```python
from build123d import *

# Parameters (mm, degrees)
Y_KSEKLIK_EKSTR_ZYON1_DEPTH = 3
Y_KSEKLIK_EKSTR_ZYON3_DEPTH = 15.352247347
KES_EKSTR_ZYON6_DEPTH       = 83.869457244
RADYUS1_R                   = 1
IZIM9_R                     = 2.8
KES_EKSTR_ZYON7_DEPTH       = 13


with BuildPart() as part:
    # Çizim1 → Yükseklik-Ekstrüzyon1 (new body)
    with BuildSketch(Plane.XY):
        with BuildLine():
            Line((51.744165627, 14.308045798), (56.895737739, 14.308045798))
            Line((56.895737739, 14.308045798), (56.895737739, 29.660293145))
            Line((56.895737739, 29.660293145), (-67.032214562, 29.660293145))
            Line((-67.032214562, 29.660293145), (-67.032214562, -18.6200596))
            add(Edge.make_bspline(
                [(51.744165627, 14.308045798), (32.353014477, 13.942055171), (-5.53549701, 3.029288221), (-42.761336594, -18.994069798), (-67.032214562, -18.6200596)],
                knots=[0, 0, 0, 0, 0.428556307, 1, 1, 1, 1], degree=3))
        make_face()
    extrude(amount=Y_KSEKLIK_EKSTR_ZYON1_DEPTH)

    # Çizim5 → Yükseklik-Ekstrüzyon3 (add)
    with BuildSketch(Plane(origin=(0, 29.660293145, 0), x_dir=(1, 0, 0), z_dir=(0, 1, 0))):
        with BuildLine():
            Line((57.574880058, 1.015986664), (56.895737739, 0))
            Line((56.895737739, 0), (56.895737739, -3))
            Line((56.895737739, -3), (57.574880058, -4.015986664))
            Line((57.574880058, -4.015986664), (57.918910072, -4.530650376))
            ThreePointArc((57.918910072, -4.530650376), (66.895737739, -1.5), (57.918910072, 1.530650376))
            Line((57.918910072, 1.530650376), (57.574880058, 1.015986664))
        make_face()
    extrude(amount=-Y_KSEKLIK_EKSTR_ZYON3_DEPTH)

    # Çizim7 → Kes-Ekstrüzyon6 (cut, through all)
    with BuildSketch(Plane(origin=(0, 29.660293145, 0), x_dir=(1, 0, 0), z_dir=(0, 1, 0))):
        Polygon((-67.032214562, -0.5), (56.895737739, 0), (-67.032214562, 0), align=None)
        Polygon((-67.032214562, -3), (56.895737739, -3), (-67.032214562, -2.5), align=None)
    extrude(amount=-KES_EKSTR_ZYON6_DEPTH, mode=Mode.SUBTRACT)

    # Radyus1
    radyus1_edges = [part.edges().sort_by_distance(p)[0] for p in [
        (-67.032214562, 5.520116772, 2.5),
        (-67.032214562, 5.520116772, 0.5),
    ]]
    fillet(radyus1_edges, radius=RADYUS1_R)

    # Çizim9 → Kes-Ekstrüzyon7 (cut)
    with BuildSketch(Plane(origin=(0, 29.660293145, 0), x_dir=(-1, 0, 0), z_dir=(0, 1, 0))):
        with Locations(Location((-61.895737739, 1.5, 0), (0, 0, 90))):
            Circle(IZIM9_R)
    extrude(amount=-KES_EKSTR_ZYON7_DEPTH, mode=Mode.SUBTRACT)


solid = part.part
```
For this review, take the finished solid that the model builds, in its own axes (mm). A direction names the side the tool comes from. Round coordinates to 2 decimals unless told otherwise and drop trailing zeros. One line per item, written item: value. Start each with the question number.
(1) Insertion check: pin 1 (1.5 mm diameter, centred on x = -4, y = 15.5, fed in from +Z); pin 2 (8 mm diameter, centred on x = -30, y = -6.5, fed in from +Z); pin 3 (1.5 mm diameter, centred on y = 23.5, z = 4.5, fed in from -X). Each pin has a flat end and moves straight along its axis. Give the tip position at first contact, or say it passes through.
(2) Machinability: for faces 1 (the flat face through (61, 14.308, 1)), 2 (the cylindrical face through (64.257, 23.251, 3.005)), which of the approach directions +Z, -Z, +X, -X, +Y, -Y give a long, thin tool a straight path to every point of the face, cutting with its end or side? Answer none if there is none.
(3) The part is to be moulded in two halves that separate along Z. For faces 3 (the flat face through (62, 16.66, 1)), 4 (the flat face through (10, 29.66, 1)), 5 (the cylindrical face through (66.893, 22.092, 1.674)), say which applies: released by +Z, released by -Z, zero draft, split by the parting line, or undercut.
(4) Wall thickness on line 1 (X direction, y = 25.5, z = 1.5); line 2 (Z direction, x = -60, y = 3); line 3 (Z direction, x = -45.5, y = 15): over which ranges is each line inside the solid? List them lowest first.
Result:
1. pin 1: z = 2.76
1. pin 2: z = 2.67
1. pin 3: x = 57.4
2. face 1: +Z, -Z, +X, -Y
2. face 2: +Y
3. face 3: undercut
3. face 4: zero draft
3. face 5: split by the parting line
4. line 1: -67.03 to 59.1, 64.7 to 66.9
4. line 2: 0.47 to 2.53
4. line 3: 0.41 to 2.59
